Can you work these out from the drawing? Everything is in mm from the part's minimum corner. A direction names the side the tool comes from. Round coordinates to 2 decimals unless told otherwise and drop trailing zeros. Loops run counter-clockwise (first coordinate to the right, second up) from the corner with the lowest first, then second, coordinate; pieces in that order, holes last. Notation, with made-up numbers: (11, -26.75) -> (15, -26.75) arc R32 ccw to (15, -0.75) -> close; hole circle Ø1 at (54, 1.5). An arc over 180 degrees is marked (long way). One line per item, written item: value.
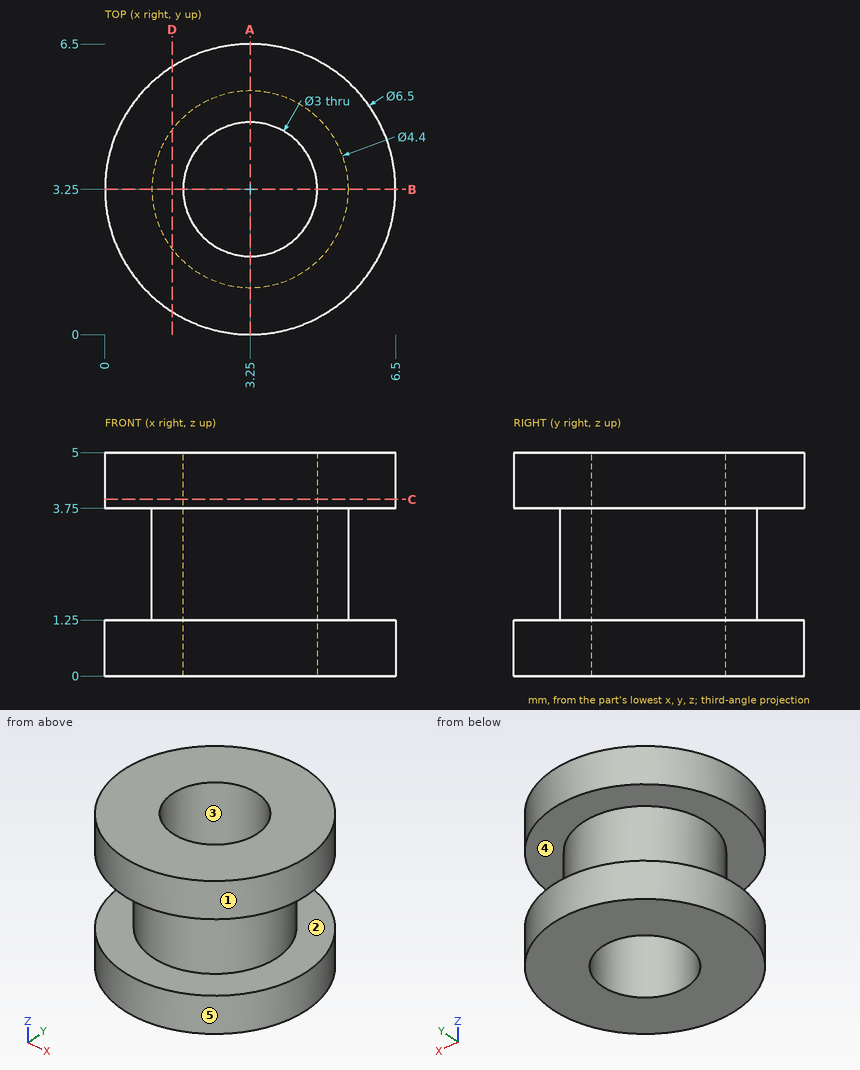
(1) For pin 1 Ø1 at (y, z) = (4.5, 2) entering from -X; pin 2 Ø1.5 at (y, z) = (2, 3.5) entering from +X; pin 3 Ø3 at (x, y) = (4, 4) entering from -Z, each with a flat end and sliding along its axis, tell me the tip position at first contact or that it passes through.
Results below:
pin 1: stops at x = 1.18
pin 2: stops at x = 6.45
pin 3: stops at z = 0
(2) Imagine slicing it at A-A on x = 3.25. Write out the boundary of the cut face in (y, z).
Results below:
outline: (0, 0) -> (1.75, 0) -> (1.75, 5) -> (0, 5) -> (0, 3.75) -> (1.05, 3.75) -> (1.05, 1.25) -> (0, 1.25) -> close; (4.75, 0) -> (6.5, 0) -> (6.5, 1.25) -> (5.45, 1.25) -> (5.45, 3.75) -> (6.5, 3.75) -> (6.5, 5) -> (4.75, 5) -> close
(3) We'd pull the mould along X, two halves only. Please class the marked faces 1, 2 and 3: +X half, -X half, draft (parallel to the pull), parting line (faces both ways), or undercut.
Results below:
face 1: parting line
face 2: draft
face 3: undercut
(4) Imagine slicing it at C-C on z = 3.95. Write out the boundary of the cut face in (x, y).
Results below:
outline: circle Ø6.5 at (3.25, 3.25); hole circle Ø3 at (3.25, 3.25)
(5) Imagine slicing it at D-D on x = 1.5. Write out the boundary of the cut face in (y, z).
Results below:
outline: (0.51, 0) -> (5.99, 0) -> (5.99, 1.25) -> (4.58, 1.25) -> (4.58, 3.75) -> (5.99, 3.75) -> (5.99, 5) -> (0.51, 5) -> (0.51, 3.75) -> (1.92, 3.75) -> (1.92, 1.25) -> (0.51, 1.25) -> close
(6) Please list where these lines run through material, in increasing order: L1, parallel to Y at x = 3.25, z = 2.1; L2, parallel to Z at x = 6, y = 1.75; L3, parallel to Y at x = 3.25, z = 0.8.
Results below:
L1: y = 1.05 to 1.75, 4.75 to 5.45
L2: z = 0 to 1.25, 3.75 to 5
L3: y = 0 to 1.75, 4.75 to 6.5
(7) On a 3-axis mill with a long thin cutter (end or side, diameter ignored), from which of +Z, -Z, +X, -X, +Y, -Y can I reach the whole of each face in a straight line? I mean the marked faces 4 and 5. Say none if no direction works.
Results below:
face 4: none
face 5: +Z, -Z
